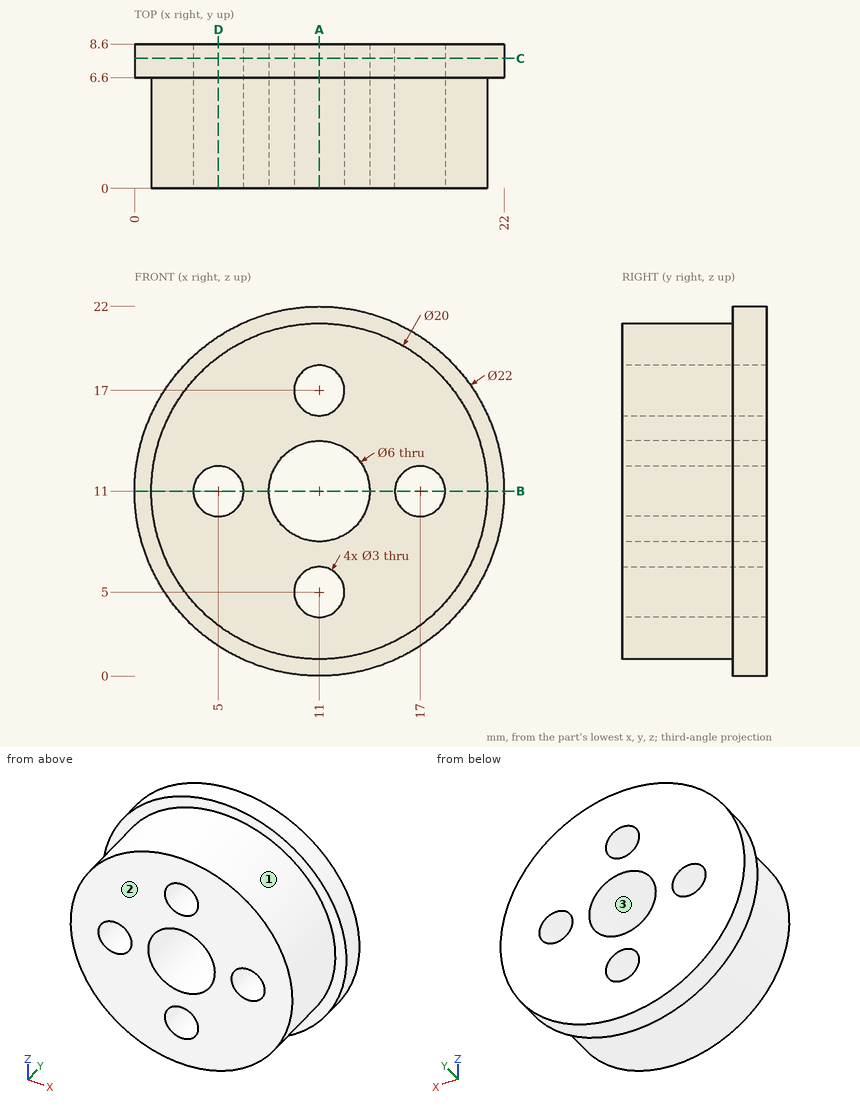
For this review, use the dimensioned drawing (mm, ordinates from the lowest corner) and the shaded views. Round coordinates to 2 decimals unless told otherwise and drop trailing zeros. Write each loop counter-clockwise with the first axis right and the second up, starting at its lowest first coordinate (ties: lowest second). Pieces come first, ordered by that corner, then holes. Notation, with made-up numbers: (-19.75, 26) -> (26.25, 26) arc R18 cw to (26.25, 34) -> close; hole circle Ø7 at (82.25, 33.5). An arc over 180 degrees is marked (long way). Use CSV: the item, a comma, the result in double quotes.
(1) To check wall thickness, follow L1, parallel to X at y = 7, z = 9.75; L2, parallel to X at y = 6.5, z = 10.5; L3, parallel to Y at x = 2, z = 16.5. State the ranges of each line that lie inside material, in increasing order. Write a range as [from, to].
Computed values:
L1,"[0.07, 4.17], [5.83, 8.27], [13.73, 16.17], [17.83, 21.93]"
L2,"[1.01, 3.59], [6.41, 8.04], [13.96, 15.59], [18.41, 20.99]"
L3,"[6.6, 8.6]"
(2) Clearance check with flat-ended pins moving along their axes: P1, Ø1.8, axis at x = 5, z = 11, coming from the -Y side; P2, Ø1.5, axis at x = 6.5, y = 2, coming from the -Z side; P3, Ø4, axis at y = 7, z = 14.5, coming from the -X side; P4, Ø1, axis at x = 12.5, y = 7, coming from the +Z side. State where each tip first meets the part, or that it passes through.
Computed values:
P1,"through"
P2,"z = 1.73"
P3,"x = 0.1"
P4,"z = 21.95"
(3) Consider section C-C, the plane y = 7.75. Give the boundary of the cut face in (x, z), plus the area to 3 significant figures.
Computed values:
outline,"circle Ø22 at (11, 11); hole circle Ø3 at (5, 11); hole circle Ø6 at (11, 11); hole circle Ø3 at (11, 5); hole circle Ø3 at (11, 17); hole circle Ø3 at (17, 11)"
area,"324 mm²"
(4) Draft analysis for pull direction Z (two halves, no side actions). For the marked faces 1, 2 and 3, state which applies: +Z half, -Z half, draft (parallel to the pull), parting line (faces both ways), or undercut.
Computed values:
face 1,"parting line"
face 2,"draft"
face 3,"undercut"
(5) Consider section D-D, the plane x = 5. Give the boundary of the cut face in (y, z), plus the area to 3 significant figures.
Computed values:
outline,"(0, 3) -> (6.6, 3) -> (6.6, 1.78) -> (8.6, 1.78) -> (8.6, 9.5) -> (0, 9.5) -> close; (0, 12.5) -> (8.6, 12.5) -> (8.6, 20.22) -> (6.6, 20.22) -> (6.6, 19) -> (0, 19) -> close"
area,"117 mm²"
(6) Consider section A-A, the plane x = 11. Give the boundary of the cut face in (y, z).
Computed values:
outline,"(0, 1) -> (6.6, 1) -> (6.6, 0) -> (8.6, 0) -> (8.6, 3.5) -> (0, 3.5) -> close; (0, 6.5) -> (8.6, 6.5) -> (8.6, 8) -> (0, 8) -> close; (0, 14) -> (8.6, 14) -> (8.6, 15.5) -> (0, 15.5) -> close; (0, 18.5) -> (8.6, 18.5) -> (8.6, 22) -> (6.6, 22) -> (6.6, 21) -> (0, 21) -> close"
(7) Consider section B-B, the plane z = 11. Give the boundary of the cut face in (x, y), plus the area to 3 significant figures.
Computed values:
outline,"(0, 6.6) -> (1, 6.6) -> (1, 0) -> (3.5, 0) -> (3.5, 8.6) -> (0, 8.6) -> close; (6.5, 0) -> (8, 0) -> (8, 8.6) -> (6.5, 8.6) -> close; (14, 0) -> (15.5, 0) -> (15.5, 8.6) -> (14, 8.6) -> close; (18.5, 0) -> (21, 0) -> (21, 6.6) -> (22, 6.6) -> (22, 8.6) -> (18.5, 8.6) -> close"
area,"72.8 mm²"
